Source: CAD feature listing. Evaluate the final solid. Frame: model axes, mm. A direction names the side the tool comes from. Coordinates: 2 decimals unless noted, no trailing zeros. Loops run counter-clockwise (first coordinate to the right, second up) from the corner with the lowest first, then second, coordinate; pieces in that order, holes last. Notation, with made-up numbers: M 59,-7.75 L 87,-7.75 A25 ccw 87,14.25 Z; hole C 52.5,21 d8. An arc over 180 degrees is marked long. One line per question, with ' | ' between items. Start each with the question number.
1. Section query B-B, the plane y = 0. Output: boundary loops of the cut face in (x, z).
2. Section query A-A, the plane x = 0. Output: boundary loops of the cut face in (y, z).
3. Section query C-C, the plane x = 36. Output: boundary loops of the cut face in (y, z).
4. Ray query, probe 1 along Y at (x, z) = (0, 3); probe 2 along Z at (x, y) = (21, 4.5); probe 3 along X at (y, z) = (2, -1.25). Return the intervals inside material, ascending.
5. Pin query (flat end, axial travel): P1, Ø1.2, axis at x = 36.5, z = -1.5, coming from the -Y side; P2, Ø2, axis at x = 30, y = -0.5, coming from the -Z side; P3, Ø4.5, axis at y = 0, z = -3, coming from the -X side. Return the tip coordinate at first contact, or that it passes through.
6. Access query for faces 4 (the flat face through (38, 5, -2)), 5 (the flat face through (34, 0, -2)), 6 (the flat face through (17, 0, 8)), 7 (the flat face through (-8, 0, 4)), 8 (the flat face through (38, -5, -2)). Directions: +Z, -Z, +X, -X, +Y, -Y. A direction counts if a zero-diameter tool reaches every point of the face in a straight line with its end or side. Return the directions, or none.
7. Mould query, pull axis X, two halves, no side actions, for faces 1 (the flat face through (38, 0, -4)), 2 (the cylindrical face through (-0.585, -2.636, 3.944)), 3 (the flat face through (42, 0, 3)). Classes: pulls with the +X half, pulls with the -X half, needs draft (parallel to the pull), parting line crosses it, or undercut.
8. Section query D-D, the plane z = 2.25. Output: boundary loops of the cut face in (x, y), and give its area (3 significant figures).
```python
from build123d import *

# Parameters (mm, degrees)
SKETCH2_W                  = 50
SKETCH2_H                  = 16
CLAMP_ARM_DEPTH            = 8
SKETCH3_R                  = 2.7
PIVOT_BOLT_CLEARANCE_DEPTH = 8
CONTACT_NOSE_START         = -4
SKETCH4_W                  = 8
SKETCH4_H                  = 10
CONTACT_NOSE_DEPTH         = 4


with BuildPart() as part:
    # Sketch2 → Clamp_arm (new body)
    with BuildSketch(Plane.XY):
        with Locations((17, 0)):
            Rectangle(SKETCH2_W, SKETCH2_H)
    extrude(amount=CLAMP_ARM_DEPTH)

    # Sketch3 → Pivot_bolt_clearance (cut)
    with BuildSketch(Plane.XY):
        Circle(SKETCH3_R)
    extrude(amount=PIVOT_BOLT_CLEARANCE_DEPTH, mode=Mode.SUBTRACT)

    # Sketch4 → Contact_nose (add)
    with BuildSketch(Plane.XY.offset(CONTACT_NOSE_START)):
        with Locations((38, 0)):
            Rectangle(SKETCH4_W, SKETCH4_H)
    extrude(amount=CONTACT_NOSE_DEPTH)


solid = part.part
```
Taken from the geometry:
1) outline: M -8,0 L -2.7,0 L -2.7,8 L -8,8 Z; M 2.7,0 L 34,0 L 34,-4 L 42,-4 L 42,8 L 2.7,8 Z
2) outline: M -8,0 L -2.7,0 L -2.7,8 L -8,8 Z; M 2.7,0 L 8,0 L 8,8 L 2.7,8 Z
3) outline: M -8,0 L -5,0 L -5,-4 L 5,-4 L 5,0 L 8,0 L 8,8 L -8,8 Z
4) probe 1: -8 to -2.7, 2.7 to 8 | probe 2: 0 to 8 | probe 3: 34 to 42
5) P1: y = -5 | P2: z = 0 | P3: x = 34
6) face 4: -Z, +X, -X, +Y | face 5: -Z, -X, +Y, -Y | face 6: +Z, +X, -X, +Y, -Y | face 7: +Z, -Z, -X, +Y, -Y | face 8: -Z, +X, -X, -Y
7) face 1: needs draft | face 2: undercut | face 3: pulls with the +X half
8) outline: M -8,-8 L 42,-8 L 42,8 L -8,8 Z; hole C 0,0 d5.4 | area: 777 mm^2
